Autodesk Inventor part; units mm, degrees
ref_plane "YZ Plane" through (0, 0, 0) normal (1, 0, 0) x (0, 1, 0)
ref_plane "XZ Plane" through (0, 0, 0) normal (0, 1, 0) x (-1, 0, 0)
ref_plane "XY Plane" through (0, 0, 0) normal (0, 0, 1) x (1, 0, 0)
sketch "Sketch1" plane through (0, 0, 0) normal (0, 1, 0) x (-1, 0, 0)
  line L0 (-20, 46) -> (20, 46)
  line L1 (20, 46) -> (20, -46)
  line L2 (20, -46) -> (-20, -46)
  line L3 (-20, -46) -> (-20, 46)
  line L4 (-20, 46) -> (20, -46) construction
  line L5 (20, 46) -> (-20, -46) construction
  point P0 (0, 0)
  dimension "d0" = 40
  dimension "d1" = 92
extrude "Extrusion1" add sketch "Sketch1" along normal blind 20
sketch "Sketch2" plane through (0, 20, 0) normal (0, 1, 0) x (1, 0, 0)
  line L0 (-20, 46) -> (-20, -46)
  line L1 (20, -46) -> (20, 46)
  line L2 (-20, -46) -> (20, -46)
  line L3 (20, -46) -> (20, 44)
  line L4 (20, 44) -> (-20, 44)
  line L5 (-20, 44) -> (-20, -46)
  point P0 (0, 0)
  point P1 (-20, 44)
  dimension "d4" = 90
extrude "Extrusion2" cut sketch "Sketch2" against normal blind 4
sketch "Sketch3" plane through (0, 16, 0) normal (0, 1, 0) x (1, 0, 0)
  line L0 (0.25, 43) -> (17.75, 43)
  line L1 (17.75, 43) -> (17.75, -27)
  line L2 (17.75, -27) -> (0.25, -27)
  line L3 (0.25, -27) -> (0.25, 43)
  line L4 (20, 44) -> (20, -46)
  line L5 (-20, 44) -> (20, 44)
  line L6 (-17.75, -27) -> (-0.25, -27)
  line L7 (-0.25, -27) -> (-0.25, 43)
  line L8 (-0.25, 43) -> (-17.75, 43)
  line L9 (-17.75, 43) -> (-17.75, -27)
  line L10 (-20, -46) -> (-20, 44)
  point P0 (0, 0)
  dimension "d7" = 17.5
  dimension "d8" = 70
  dimension "d9" = 2.25
  dimension "d10" = 1
  dimension "d11" = 17.5
  dimension "d12" = 2.25
  dimension "d13" = 1
extrude "Extrusion3" cut sketch "Sketch3" against normal blind 7
sketch "Sketch4" plane through (0.25, 16, 27) normal (1, 0, 0) x (0, 0, -1)
  line L0 (0, 0) -> (70, 0)
  line L1 (14.131, 0) -> (17.5, -3.369)
  line L2 (17.5, -3.369) -> (52.5, -3.369)
  line L3 (70, 0) -> (0, 0)
  line L4 (52.5, -3.369) -> (55.869, 0)
  line L5 (0, 0) -> (0, -7)
  line L6 (70, 0) -> (70, -7)
  point P0 (27, -16)
  point P1 (0, -3.5)
  point P2 (70, -3.5)
  dimension "d16" = 45
  dimension "d17" = 45
  dimension "d18" = 17.5
  dimension "d19" = 17.5
extrude "Extrusion4" cut sketch "Sketch4" against normal up to surface (0.5 mm away)
fillet "Fillet1" radius 2.5 2 edges at (20, 20, -45) (-20, 20, -45)
sketch "Sketch5" plane through (0, 16, 0) normal (0, 1, 0) x (1, 0, 0)
  line L0 (20, 44) -> (20, -46)
  line L1 (-20, 44) -> (20, 44)
  line L2 (20, 44) -> (20, -46)
  line L3 (20, -46) -> (-20, -46)
  line L4 (-20, -46) -> (-20, 44)
  line L5 (-19.5, 44.1346) -> (19.5, 44.1346)
  line L6 (19.5, 44.1346) -> (19.5, -45.5)
  line L7 (19.5, -45.5) -> (-19.5, -45.5)
  line L8 (-19.5, -45.5) -> (-19.5, 44.1346)
  line L9 (-17.75, 43) -> (-0.25, 43)
  point P0 (0, 0)
  point P1 (19.5, 44)
  point P2 (-19.5, 44)
  dimension "d23" = 0.5
  dimension "d24" = 0.5
  dimension "d25" = 0.5
extrude "Extrusion5" cut sketch "Sketch5" against normal blind 0.5 contours L0 L3 L4 L1 L8 L7 L6
properties part number "Battery Pack 9.2x4" material "PC/ABS Plastic"
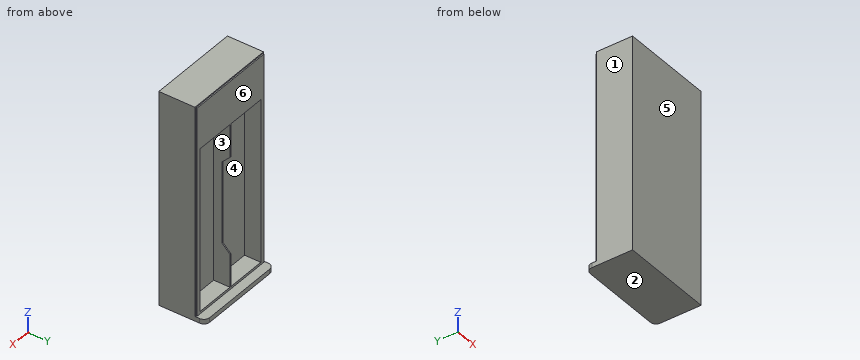
The model under review builds one solid part; all positions refer to its coordinate system, in mm. Face numbers are marked on the shaded views. A direction names the side the tool comes from. Give positions to 0.01 mm unless a question says otherwise; leave off trailing zeros. Write each loop counter-clockwise with the first axis right and the second up, starting at its lowest first coordinate (ties: lowest second). Pieces come first, ordered by that corner, then holes. Notation, with made-up numbers: M 73,53.25 L 121,53.25 A14 ccw 121,66.25 Z; hole C 30.25,-22 d9. An arc over 180 degrees is marked long. Write each question's results on one line, items separated by ' | '. Start each with the question number.
1. Insertion check: pin 1 Ø10 at (y, z) = (16.5, -2) entering from -X; pin 2 Ø2 at (x, z) = (-16, 35) entering from +Y; pin 3 Ø5 at (x, z) = (-5.5, 4.5) entering from +Y; pin 4 Ø0.6 at (x, z) = (0, -9) entering from +Y. Each pin has a flat end and moves straight along its axis. Give the tip position at first contact, or say it passes through.
2. For probe 1 along X at (y, z) = (10.5, -36); probe 2 along Z at (x, y) = (7, 10.25); probe 3 along Y at (x, z) = (5, -41), list the stretches that pass through material, from the lowest coordinate up. Write a range as [from, to].
3. We need section A-A (z = 38.5). Write out the cut boundary in (x, y), and give its area (4 significant figures).
4. We need section D-D (z = 26). Write out the cut boundary in (x, y).
5. For the marked faces 4, 5 and 6, list the 3-axis set-ups (+Z, -Z, +X, -X, +Y, -Y) from which the entire face can be reached by the end or side of a thin tool; tool diameter is ignored.
6. Mouldability with a two-part tool opening along X and no side actions: class the marked faces 1, 2 and 3 as released by +X, released by -X, zero draft, split by the parting line, or undercut.
7. We need section C-C (y = 11.75). Write out the cut boundary in (x, z).
8. We need section B-B (x = 13). Write out the cut boundary in (y, z).
Results found:
1) pin 1: stops at x = -20 | pin 2: stops at y = 16 | pin 3: stops at y = 9 | pin 4: stops at y = 12.63
2) probe 1: x = [-20, -17.75], [-0.25, 0.25], [17.75, 20] | probe 2: z = [-46, -43], [27, 46] | probe 3: y = [0, 9]
3) outline: M -20,0 L 20,0 L 20,15.5 L 19.5,15.5 L 19.5,16 L -19.5,16 L -19.5,15.5 L -20,15.5 Z | area: 639.5 mm^2
4) outline: M -20,0 L 20,0 L 20,15.5 L 19.5,15.5 L 19.5,16 L 17.75,16 L 17.75,9 L 0.25,9 L 0.25,16 L -0.25,16 L -0.25,9 L -17.75,9 L -17.75,16 L -19.5,16 L -19.5,15.5 L -20,15.5 Z
5) face 4: +Y | face 5: +Z, -Z, +X, -X, -Y | face 6: +Z, +X, -X, +Y
6) face 1: released by -X | face 2: zero draft | face 3: undercut
7) outline: M -20,-46 L 20,-46 L 20,46 L -20,46 Z; hole M -17.75,-43 L -0.25,-43 L -0.25,27 L -17.75,27 Z; hole M 0.25,-43 L 17.75,-43 L 17.75,27 L 0.25,27 Z
8) outline: M 0,-46 L 20,-46 L 20,-44 L 16,-44 L 16,-43 L 9,-43 L 9,27 L 16,27 L 16,45.5 L 15.5,45.5 L 15.5,46 L 0,46 Z
